```python
from build123d import *

# Parameters (mm, degrees)
F0_W     = 94.0314047039
F0_H     = 61.6279765964
F0_W_2   = 7.300876081
F0_H_2   = 0.858925283
F1_DEPTH = 25.4
F2_DEPTH = 12.7


with BuildPart() as f1:
    # F0 (on Front) → F1 (new body)
    with BuildSketch(Plane.XZ):
        Polygon((-130.7592019439, -35.8140021563), (38.1000041962, -35.8140021563), (38.1000041962, 138.5316029191), (-36.72779724, 138.5316029191), (-36.72779724, 76.9036263227), (-130.7592019439, 76.9036263227), align=None)
        Polygon((-138.9400362968, 76.9036263227), (-130.7592019439, 76.9036263227), (-130.7592019439, 138.5316029191), (-36.72779724, 138.5316029191), (-36.72779724, 142.6114886999), (-138.9400362968, 142.6114886999), align=None)
        with Locations((-83.7434995919, 107.7176146209)):
            Rectangle(F0_W, F0_H)
        with Locations((-84.6129395068, 94.9410833418)):
            Rectangle(F0_W_2, F0_H_2, mode=Mode.SUBTRACT)
    extrude(amount=F1_DEPTH)

    # F2 (cut, symmetric): a face of the model
    f2_faces = [f1.faces().sort_by_distance(p)[0] for p in [
        (-48.3621229952, -25.4, 53.5114771405),
    ]]
    extrude(f2_faces, amount=F2_DEPTH, both=True, mode=Mode.SUBTRACT)


solid = f1.part
```
Verification items for the finished model (mm, model axes). A direction names the side the tool comes from. Give positions to 0.01 mm unless a question says otherwise; leave off trailing zeros. Loops run counter-clockwise (first coordinate to the right, second up) from the corner with the lowest first, then second, coordinate; pieces in that order, holes last. Notation, with made-up numbers: M 63,45.25 L 105,45.25 A28 ccw 105,83.25 Z; hole C 61,21 d4. An arc over 180 degrees is marked long. Return JSON: item names as keys, results as strings.
1) Gauge pin test, flat ends, axial feed: P1, Ø2, axis at x = 2, y = -10, coming from the +Z side; P2, Ø2, axis at y = -5, z = 141.5, coming from the +X side; P3, Ø2.5, axis at x = -135, y = -4, coming from the -Z side. Record the tip position at first contact, or that the pin passes through.
Findings:
{"P1": "stops at z = 138.53", "P2": "stops at x = -36.73", "P3": "stops at z = 76.9"}
2) Tool access check on faces 1 (the flat face through (-36.728, -6, 141)), 2 (the flat face through (-85, -6, 94.512)), 3 (the flat face through (-135, -6, 76.904)). Record the directions out of +Z, -Z, +X, -X, +Y, -Y that give a thin tool (end or side, any length) a straight path to the whole face; none if there is none.
Findings:
{"face 1": "+Z, +X, +Y, -Y", "face 2": "+Y, -Y", "face 3": "-Z, -X, +Y, -Y"}
3) Section check C-C, the plane z = 74. Enter the section's corners in (x, y).
Findings:
{"outline": "M -130.76,-12.7 L 38.1,-12.7 L 38.1,0 L -130.76,0 Z"}
4) Section check A-A, the plane y = -5.75. Enter the section's corners in (x, z), and give its area (3 significant figures).
Findings:
{"outline": "M -138.94,76.9 L -130.76,76.9 L -130.76,-35.81 L 38.1,-35.81 L 38.1,138.53 L -36.73,138.53 L -36.73,142.61 L -138.94,142.61 Z; hole M -88.26,94.51 L -80.96,94.51 L -80.96,95.37 L -88.26,95.37 Z", "area": "30,400 mm2"}
5) Material ranges on L1, parallel to X at y = -8, z = -21.5; L2, parallel to Z at x = -27, y = -6.75, recorded low to high. Write a range as [from, to].
Findings:
{"L1": "x = [-130.76, 38.1]", "L2": "z = [-35.81, 138.53]"}
6) Mould release check, pull along X, two halves, no side actions. Record for faces 4 (the flat face through (-85, -6, 95.371)), 5 (the flat face through (38.1, -6, 50)), 6 (the flat face through (-52, -12.7, 55)): released by +X, released by -X, zero draft, split by the parting line, or undercut.
Findings:
{"face 4": "undercut", "face 5": "released by +X", "face 6": "zero draft"}
7) Section check B-B, the plane x = 25. Enter the section's corners in (y, z), and give its area (3 significant figures).
Findings:
{"outline": "M -12.7,-35.81 L 0,-35.81 L 0,138.53 L -12.7,138.53 Z", "area": "2,210 mm2"}
